from build123d import *

# Parameters (mm, degrees)
SKETCH1_W           = 20
SKETCH1_H           = 20
SKETCH1_W_2         = 75
SKETCH1_H_2         = 25
BOSS_EXTRUDE1_DEPTH = 10
CUT_EXTRUDE1_REACH  = 52.621
SKETCH2_R           = 3.5
SKETCH2_R_2         = 4.35
FILLET1_R           = 5
SKETCH3_R           = 6
CUT_EXTRUDE2_DEPTH  = 4


with BuildPart() as part:
    # Sketch1 → Boss-Extrude1 (new body)
    with BuildSketch(Plane(origin=(0, 0, 0), x_dir=(1, 0, 0), z_dir=(0, 1, 0))):
        with Locations((27.5, 22.5)):
            Rectangle(SKETCH1_W, SKETCH1_H)
        Rectangle(SKETCH1_W_2, SKETCH1_H_2)
        with Locations((27.5, -22.5)):
            Rectangle(SKETCH1_W, SKETCH1_H)
    extrude(amount=BOSS_EXTRUDE1_DEPTH)

    # Sketch2 → Cut-Extrude1 (cut, up to next)
    with BuildSketch(Plane(origin=(0, 10, 0), x_dir=(1, 0, 0), z_dir=(0, 1, 0)), mode=Mode.PRIVATE) as cut_extrude1_sk1:
        with Locations(Location((-25.5, 0, 0), (0, 0, 270))):
            Circle(SKETCH2_R)
    cut_extrude1_tool1 = extrude(cut_extrude1_sk1.sketch, amount=-CUT_EXTRUDE1_REACH, mode=Mode.PRIVATE) & part.part
    # Sketch2 → Cut-Extrude1 (cut, up to next)
    with BuildSketch(Plane(origin=(0, 10, 0), x_dir=(1, 0, 0), z_dir=(0, 1, 0)), mode=Mode.PRIVATE) as cut_extrude1_sk2:
        with Locations(Location((27.5, 0, 0), (0, 0, 270))):
            Circle(SKETCH2_R_2)
    cut_extrude1_tool2 = extrude(cut_extrude1_sk2.sketch, amount=-CUT_EXTRUDE1_REACH, mode=Mode.PRIVATE) & part.part
    add(cut_extrude1_tool1.solids().sort_by_distance((-25.5, 10, 0))[0], mode=Mode.SUBTRACT)
    add(cut_extrude1_tool2.solids().sort_by_distance((27.5, 10, 0))[0], mode=Mode.SUBTRACT)

    # Fillet1
    fillet1_edges = [part.edges().sort_by_distance(p)[0] for p in [
        (17.5, 5, -32.5),
        (37.5, 5, -32.5),
        (37.5, 5, 32.5),
        (17.5, 5, 32.5),
        (17.5, 5, 12.5),
        (-37.5, 5, 12.5),
        (-37.5, 5, -12.5),
        (17.5, 5, -12.5),
    ]]
    fillet(fillet1_edges, radius=FILLET1_R)

    # Sketch3 → Cut-Extrude2 (cut)
    with BuildSketch(Plane.XZ):
        with Locations(Location((-25.5, 0, 0), (0, 0, 270))):
            Circle(SKETCH3_R)
    extrude(amount=-CUT_EXTRUDE2_DEPTH, mode=Mode.SUBTRACT)


solid = part.part
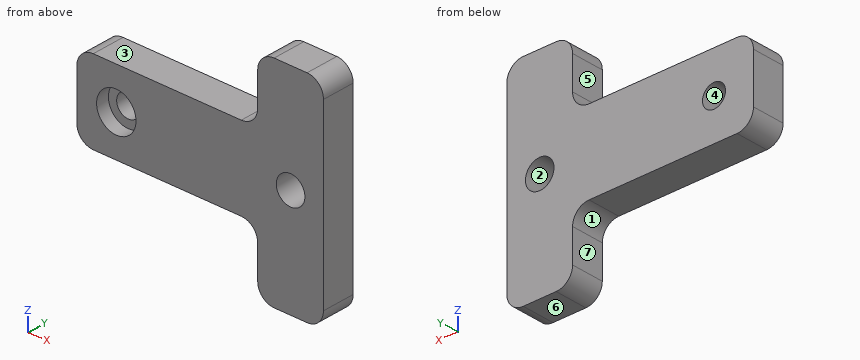
Check sheet for the modelled part. Datum: model origin and axes. Units: mm. Face numbers are marked on the shaded views. A direction names the side the tool comes from. Round coordinates to 2 decimals unless told otherwise and drop trailing zeros. Write each loop counter-clockwise with the first axis right and the second up, starting at its lowest first coordinate (ties: lowest second). Pieces come first, ordered by that corner, then holes. Notation, with made-up numbers: (5.5, 16) -> (24.5, 16) arc R13 cw to (24.5, 29) -> close; hole circle Ø2 at (-39.5, -15.5). An arc over 180 degrees is marked (long way). Answer as CSV lines item,"result". Start each with the question number.
1) Release check for a two-part mould opening along X. For the marked faces 1, 2, 3 and 4 record: pulls with the +X half, pulls with the -X half, needs draft (parallel to the pull), parting line crosses it, or undercut.
2) Section check C-C on y = 7.5. Enter the section's corners in (x, z), and give its area (3 significant figures).
3) Go/stop test with flat-tipped pins: P1, Ø8, axis at x = -25.5, z = 0, coming from the -Y side; P2, Ø8, axis at x = 27.5, z = 0, coming from the +Y side; P3, Ø6, axis at x = -1.5, y = 3.5, coming from the -Z side; P4, Ø6, axis at x = -21, y = 6, coming from the +Z side. Record where each tip stops, or that it passes through.
4) Material ranges on line 1 (X direction, y = 1.35, z = 0); line 2 (X direction, y = 7.05, z = 0); line 3 (Z direction, x = 3.5, y = 9), recorded low to high. Write a range as from..to.
5) Section check D-D on x = -25.5. Enter the section's corners in (y, z).
6) Section check A-A on z = 0. Enter the section's corners in (x, y), and give its area (3 significant figures).
7) Tool access check on the marked faces 5, 6 and 7. Record the directions out of +Z, -Z, +X, -X, +Y, -Y that give a thin tool (end or side, any length) a straight path to the whole face; none if there is none.
8) Section check B-B on x = 27.5. Enter the section's corners in (y, z).
Found:
1,face 1,"pulls with the -X half"
1,face 2,"undercut"
1,face 3,"needs draft"
1,face 4,"undercut"
2,outline,"(-37.5, -7.5) arc R5 ccw to (-32.5, -12.5) -> (12.5, -12.5) arc R5 cw to (17.5, -17.5) -> (17.5, -27.5) arc R5 ccw to (22.5, -32.5) -> (32.5, -32.5) arc R5 ccw to (37.5, -27.5) -> (37.5, 27.5) arc R5 ccw to (32.5, 32.5) -> (22.5, 32.5) arc R5 ccw to (17.5, 27.5) -> (17.5, 17.5) arc R5 cw to (12.5, 12.5) -> (-32.5, 12.5) arc R5 ccw to (-37.5, 7.5) -> close; hole circle Ø7 at (-25.5, 0); hole circle Ø8.7 at (27.5, 0)"
2,area,"2,560 mm^2"
3,P1,"stops at y = 4"
3,P2,"passes through"
3,P3,"stops at z = -12.5"
3,P4,"stops at z = 12.5"
4,line 1,"x = -37.5..-31.5, -19.5..23.15, 31.85..37.5"
4,line 2,"x = -37.5..-29, -22..23.15, 31.85..37.5"
4,line 3,"z = -12.5..12.5"
5,outline,"(0, -12.5) -> (10, -12.5) -> (10, -3.5) -> (4, -3.5) -> (4, -6) -> (0, -6) -> close; (0, 6) -> (4, 6) -> (4, 3.5) -> (10, 3.5) -> (10, 12.5) -> (0, 12.5) -> close"
6,outline,"(-37.5, 0) -> (-31.5, 0) -> (-31.5, 4) -> (-29, 4) -> (-29, 10) -> (-37.5, 10) -> close; (-22, 4) -> (-19.5, 4) -> (-19.5, 0) -> (23.15, 0) -> (23.15, 10) -> (-22, 10) -> close; (31.85, 0) -> (37.5, 0) -> (37.5, 10) -> (31.85, 10) -> close"
6,area,"573 mm^2"
7,face 5,"+Z, -X, +Y, -Y"
7,face 6,"-Z, +X, -X, +Y, -Y"
7,face 7,"-Z, -X, +Y, -Y"
8,outline,"(0, -32.5) -> (10, -32.5) -> (10, -4.35) -> (0, -4.35) -> close; (0, 4.35) -> (10, 4.35) -> (10, 32.5) -> (0, 32.5) -> close"
